Autodesk Inventor part; units mm, degrees
ref_plane "YZ Plane" through (0, 0, 0) normal (1, 0, 0) x (0, 1, 0)
ref_plane "XZ Plane" through (0, 0, 0) normal (0, 1, 0) x (-1, 0, 0)
ref_plane "XY Plane" through (0, 0, 0) normal (0, 0, 1) x (1, 0, 0)
sketch "Sketch1" plane through (0, 0, 0) normal (0, 0, 1) x (1, 0, 0)
  line L0 (0, 0) -> (25.4, 0)
  line L1 (25.4, 0) -> (25.4, 25.4)
  line L2 (25.4, 25.4) -> (0, 25.4)
  line L3 (0, 25.4) -> (0, 0)
  line L4 (3.175, 22.225) -> (22.225, 22.225)
  line L5 (22.225, 22.225) -> (22.225, 3.175)
  line L6 (22.225, 3.175) -> (3.175, 3.175)
  line L7 (3.175, 3.175) -> (3.175, 22.225)
  dimension "d0" = 25.4
  dimension "d1" = 25.4
  dimension "d2" = 3.175
extrude "Extrusion1" add sketch "Sketch1" along normal blind 609.6
sketch "Sketch2" plane through (0, 25.4, 0) normal (0, 1, 0) x (1, 0, 0)
  line L0 (22.225, 0) -> (3.175, 0) construction
  line L1 (12.7, 0) -> (12.7, -12.7) construction
  line L2 (12.7, -12.7) -> (12.7, -38.1) construction
  line L3 (0, 0) -> (0, -609.6) construction
  line L4 (0, -304.8) -> (25.4, -304.8) construction
  line L5 (25.4, 0) -> (25.4, -609.6) construction
  circle A0 centre (12.7, -38.1) radius 2.5797
  circle A1 centre (12.7, -12.7) radius 2.5797
  circle A2 centre (12.7, -571.5) radius 2.5797
  circle A3 centre (12.7, -596.9) radius 2.5797
  dimension "d5" = 12.7
  dimension "d6" = 25.4
  dimension "d7" = 5.1594
extrude "Extrusion2" cut sketch "Sketch2" against normal blind 609.6
sketch "Sketch3" plane through (25.4, 0, 0) normal (1, 0, 0) x (0, 0, -1)
  line L0 (0, 25.4) -> (-609.6, 25.4) construction
  line L1 (-304.8, 25.4) -> (-304.8, 0) construction
  line L2 (-304.8, 12.7) -> (-204.8, 12.7) construction
  line L3 (-204.8, 12.7) -> (-217.5, 12.7) construction
  line L4 (-217.5, 12.7) -> (-192.1, 12.7) construction
  circle A0 centre (-217.5, 12.7) radius 2.5797
  circle A1 centre (-192.1, 12.7) radius 2.5797
  circle A2 centre (-392.1, 12.7) radius 2.5797
  circle A3 centre (-417.5, 12.7) radius 2.5797
  point P0 (0, 0)
  dimension "d10" = 100
  dimension "d11" = 12.7
  dimension "d12" = 25.4
  dimension "d13" = 5.1594
extrude "Extrusion3" cut sketch "Sketch3" against normal blind 25.4
properties part number "2ft 1x1"
Can you work these out from the model? Positions are in its coordinate system, mm. A direction names the side the tool comes from. Coordinates: 2 decimals unless noted, no trailing zeros. Write each loop counter-clockwise with the first axis right and the second up, starting at its lowest first coordinate (ties: lowest second). Pieces come first, ordered by that corner, then holes. Notation, with made-up numbers: (12.25, 24.25) - (57.25, 24.25) arc R16 ccw to (57.25, 41.25) - close; hole circle Ø6 at (25.5, 29). An arc over 180 degrees is marked (long way). Return JSON: item names as keys, results as strings.
Q1. Please list where these lines run through material, in increasing order: L1, parallel to Z at x = 12.7, y = 0.9; L2, parallel to Y at x = 17.75, z = 289.5 (3 decimals). Write a range as from..to.
Computed values:
{"L1": "z = 0..10.12, 15.28..35.52, 40.68..568.92, 574.08..594.32, 599.48..609.6", "L2": "y = 0..3.175, 22.225..25.4"}
Q2. I'm going to push a flat-ended pin straight in: pin 1 Ø4 at (y, z) = (12.7, 417.5) entering from -X (3 decimals). Where does the tip first touch, or does it pass through?
Computed values:
{"pin 1": "passes through"}
Q3. On a 3-axis mill with a long thin cutter (end or side, diameter ignored), from which of +Z, -Z, +X, -X, +Y, -Y can I reach the whole of each face in a straight line? I mean faces 1 (the flat face through (22.225, 13, 301)), 2 (the flat face through (24, 13, 0)). Say none if no direction works.
Computed values:
{"face 1": "+Z, -Z", "face 2": "-Z, +X, -X, +Y, -Y"}
Q4. Thinking about a two-plate mould opening in X: for faces 3 (the flat face through (24, 13, 609.6)), 4 (the flat face through (25.4, 13, 301)), 5 (the flat face through (0, 13, 301)), 6 (the flat face through (13, 3.175, 301)), which applies, +X half, -X half, draft (parallel to the pull), parting line (faces both ways), or undercut?
Computed values:
{"face 3": "draft", "face 4": "+X half", "face 5": "-X half", "face 6": "undercut"}
Q5. If we section it at A-A (z = 111): Please give me the cut outline in (x, y) (3 decimals), then the cut area to 3 significant figures.
Computed values:
{"outline": "(0, 0) - (25.4, 0) - (25.4, 25.4) - (0, 25.4) - close; hole (3.175, 3.175) - (22.225, 3.175) - (22.225, 22.225) - (3.175, 22.225) - close", "area": "282 mm2"}
